from build123d import *

# Parameters (mm, degrees)
SKETCH1_W                                           = 19.05
SKETCH1_H                                           = 12.7
BOSS_EXTRUDE1_DEPTH                                 = 100
CBORE_FOR_M8_HEX_SOCKET_HEAD_CAP_SCREW1_D           = 9
CBORE_FOR_M8_HEX_SOCKET_HEAD_CAP_SCREW1_CBORE_D     = 15
CBORE_FOR_M8_HEX_SOCKET_HEAD_CAP_SCREW1_CBORE_DEPTH = 9
CHAMFER1_SIZE                                       = 1.5875


with BuildPart() as part:
    # Sketch1 → Boss-Extrude1 (new, symmetric)
    with BuildSketch(Plane(origin=(0, 0, 0), x_dir=(0, 0, -1), z_dir=(1, 0, 0))):
        Rectangle(SKETCH1_W, SKETCH1_H)
    extrude(amount=BOSS_EXTRUDE1_DEPTH, both=True)

    # CBORE for M8 Hex Socket Head Cap Screw1 (through all)
    with Locations(Plane(origin=(-66.368908966, -6.35, -4.540102203), x_dir=(1, 0, 0), z_dir=(0, -1, 0))):
        with Locations((-13.631091034, 4.540102203), (66.368908966, 4.540102203), (146.368908966, 4.540102203)):
            CounterBoreHole(CBORE_FOR_M8_HEX_SOCKET_HEAD_CAP_SCREW1_D / 2, CBORE_FOR_M8_HEX_SOCKET_HEAD_CAP_SCREW1_CBORE_D / 2, CBORE_FOR_M8_HEX_SOCKET_HEAD_CAP_SCREW1_CBORE_DEPTH)

    # Chamfer1
    chamfer1_edges = [part.edges().sort_by_distance(p)[0] for p in [
        (0, 6.35, 9.525),
        (0, 6.35, -9.525),
    ]]
    chamfer(chamfer1_edges, length=CHAMFER1_SIZE)


solid = part.part
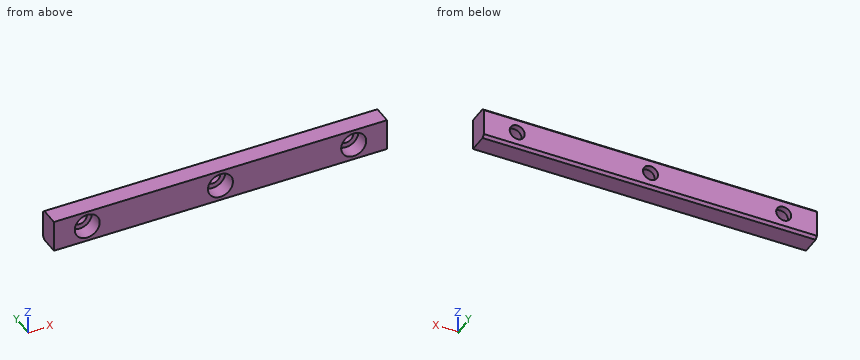
Verification items for the finished model (mm, model axes). Round coordinates to 2 decimals unless told otherwise and drop trailing zeros. Loops run counter-clockwise (first coordinate to the right, second up) from the corner with the lowest first, then second, coordinate; pieces in that order, holes last. Notation, with made-up numbers: (48.5, 82.25) - (71.5, 82.25) arc R33 cw to (71.5, 110.25) - close; hole circle Ø2 at (-8.75, -26). An arc over 180 degrees is marked (long way). Write item = value, one per line.
Q1. Sectioned sample at B-B on z = 0. Record the boundary of the cut face in (x, y).
Here are the results:
outline = (-100, -6.35) - (-87.5, -6.35) - (-87.5, 2.65) - (-84.5, 2.65) - (-84.5, 6.35) - (-100, 6.35) - close; (-75.5, 2.65) - (-72.5, 2.65) - (-72.5, -6.35) - (-7.5, -6.35) - (-7.5, 2.65) - (-4.5, 2.65) - (-4.5, 6.35) - (-75.5, 6.35) - close; (4.5, 2.65) - (7.5, 2.65) - (7.5, -6.35) - (72.5, -6.35) - (72.5, 2.65) - (75.5, 2.65) - (75.5, 6.35) - (4.5, 6.35) - close; (84.5, 2.65) - (87.5, 2.65) - (87.5, -6.35) - (100, -6.35) - (100, 6.35) - (84.5, 6.35) - close
Q2. Material ranges on L1, parallel to X at y = -4.25, z = 0.5; L2, parallel to X at y = 4.25, z = 2.75; L3, parallel to Z at x = -80, y = 4 (3 decimals), recorded low to high.
Here are the results:
L1 = -100 to -87.48, -72.52 to -7.48, 7.48 to 72.52, 87.48 to 100
L2 = -100 to -83.56, -76.44 to -3.56, 3.56 to 76.44, 83.56 to 100
L3 = -9.525 to -4.5, 4.5 to 9.525
Q3. Depth check by flat-ended pin: pin 1 (7.5 mm diameter, centred on x = 78.5, z = -3, fed in from -Y). Enter the tip coordinate at first touch or a pass-through.
Here are the results:
pin_1 = 2.65
